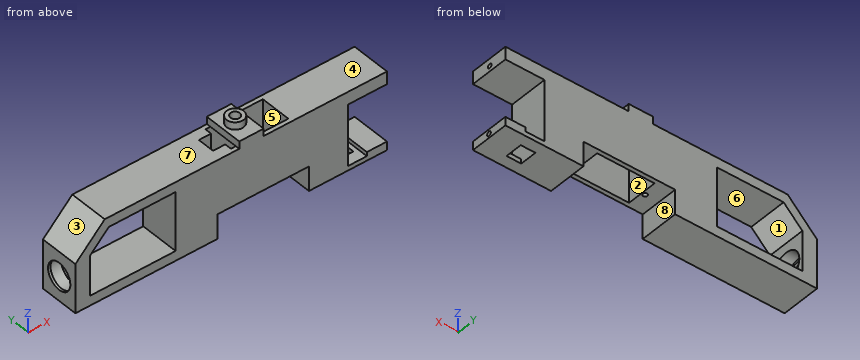
from build123d import *

# Parameters (mm, degrees)
BOSS_EXTRUDE1_DEPTH      = 8
BOSS_EXTRUDE1_DEPTH_BACK = 8
SKETCH2_R                = 5.5
CUT_EXTRUDE1_DEPTH       = 8
CUT_EXTRUDE2_DEPTH       = 16
SKETCH4_R                = 6.5
CUT_EXTRUDE3_DEPTH       = 5
SKETCH5_W                = 23.5
SKETCH5_H                = 12.6
CUT_EXTRUDE4_DEPTH       = 33
SKETCH6_R                = 0.9
CUT_EXTRUDE5_DEPTH       = 17
SKETCH7_W                = 6
SKETCH7_H                = 7
CUT_EXTRUDE6_DEPTH       = 7
SKETCH8_W                = 5
SKETCH8_H                = 7
CUT_EXTRUDE7_DEPTH       = 10
SKETCH9_R                = 0.899999999
CUT_EXTRUDE8_DEPTH       = 7
SKETCH10_W               = 37.5
SKETCH10_H               = 16
CUT_EXTRUDE9_DEPTH       = 10
SKETCH11_W               = 10
SKETCH11_H               = 16
BOSS_EXTRUDE2_DEPTH      = 3
SKETCH12_R               = 3.5
SKETCH12_R_2             = 1.9
BOSS_EXTRUDE3_DEPTH      = 3
SKETCH13_R               = 1.9
CUT_EXTRUDE10_DEPTH      = 3


with BuildPart() as part:
    # Sketch1 → Boss-Extrude1 (new body, two sides)
    with BuildSketch(Plane(origin=(0, 0, 0), x_dir=(1, 0, 0), z_dir=(0, 1, 0))) as boss_extrude1_sk:
        Polygon((64, -16.835969506), (47.993540801, -16.835969506), (47.993540801, 8.164030494), (55.763890835, 8.164030494), (55.763890835, 6.5), (64, 6.5), (64, 10), (-63.5, 10), (-63.5, -10), (-51.5, -22), (64, -22), align=None)
    extrude(amount=BOSS_EXTRUDE1_DEPTH)
    extrude(boss_extrude1_sk.sketch, amount=-BOSS_EXTRUDE1_DEPTH_BACK)

    # Sketch2 → Cut-Extrude1 (cut)
    with BuildSketch(Plane.ZY.offset(63.5)):
        Circle(SKETCH2_R)
    extrude(amount=-CUT_EXTRUDE1_DEPTH, mode=Mode.SUBTRACT)

    # Sketch3 → Cut-Extrude2 (cut)
    with BuildSketch(Plane(origin=(0, 8, 0), x_dir=(1, 0, 0), z_dir=(0, 1, 0))):
        Polygon((-57.5, 6), (-22.5, 6), (-22.5, -18), (-49.843145751, -18), (-57.5, -10.343145751), align=None)
    extrude(amount=-CUT_EXTRUDE2_DEPTH, mode=Mode.SUBTRACT)

    # Sketch4 → Cut-Extrude3 (cut)
    with BuildSketch(Plane(origin=(-57.5, 0, 0), x_dir=(0, 0, -1), z_dir=(1, 0, 0))):
        Circle(SKETCH4_R)
    extrude(amount=-CUT_EXTRUDE3_DEPTH, mode=Mode.SUBTRACT)

    # Sketch5 → Cut-Extrude4 (cut, through all)
    with BuildSketch(Plane(origin=(0, 0, -10), x_dir=(-1, 0, 0), z_dir=(0, 0, -1))):
        with Locations((-13.3, 0)):
            Rectangle(SKETCH5_W, SKETCH5_H)
    extrude(amount=-CUT_EXTRUDE4_DEPTH, mode=Mode.SUBTRACT)

    # Sketch6 → Cut-Extrude5 (cut)
    with BuildSketch(Plane(origin=(0, 0, -10), x_dir=(-1, 0, 0), z_dir=(0, 0, -1))):
        with Locations((-0.2, 0)):
            Circle(SKETCH6_R)
        with Locations((-27.5, 0)):
            Circle(SKETCH6_R)
    extrude(amount=-CUT_EXTRUDE5_DEPTH, mode=Mode.SUBTRACT)

    # Sketch7 → Cut-Extrude6 (cut)
    with BuildSketch(Plane(origin=(0, 0, -10), x_dir=(-1, 0, 0), z_dir=(0, 0, -1))):
        with Locations((-50.993540801, 0)):
            Rectangle(SKETCH7_W, SKETCH7_H)
    extrude(amount=-CUT_EXTRUDE6_DEPTH, mode=Mode.SUBTRACT)

    # Sketch8 → Cut-Extrude7 (cut)
    with BuildSketch(Plane.XY.offset(22)):
        with Locations((-0.95, 0)):
            Rectangle(SKETCH8_W, SKETCH8_H)
    extrude(amount=-CUT_EXTRUDE7_DEPTH, mode=Mode.SUBTRACT)

    # Sketch9 → Cut-Extrude8 (cut)
    with BuildSketch(Plane(origin=(64, 0, 0), x_dir=(0, 0, -1), z_dir=(1, 0, 0))):
        with Locations((-18.998394534, 0.246992199)):
            Circle(SKETCH9_R)
        with Locations((8.299298665, -0.107896588)):
            Circle(SKETCH9_R)
    extrude(amount=-CUT_EXTRUDE8_DEPTH, mode=Mode.SUBTRACT)

    # Sketch10 → Cut-Extrude9 (cut)
    with BuildSketch(Plane(origin=(0, 0, -10), x_dir=(-1, 0, 0), z_dir=(0, 0, -1))):
        with Locations((-13.3, 0)):
            Rectangle(SKETCH10_W, SKETCH10_H)
    extrude(amount=-CUT_EXTRUDE9_DEPTH, mode=Mode.SUBTRACT)

    # Sketch11 → Boss-Extrude2 (add)
    with BuildSketch(Plane.XY.offset(22)):
        with Locations((8.55, 0)):
            Rectangle(SKETCH11_W, SKETCH11_H)
    extrude(amount=BOSS_EXTRUDE2_DEPTH)

    # Sketch12 → Boss-Extrude3 (add)
    with BuildSketch(Plane.XY.offset(25)):
        with Locations((8.499999912, 0)):
            Circle(SKETCH12_R)
        with Locations((8.499999912, 0)):
            Circle(SKETCH12_R_2, mode=Mode.SUBTRACT)
    extrude(amount=BOSS_EXTRUDE3_DEPTH)

    # Sketch13 → Cut-Extrude10 (cut)
    with BuildSketch(Plane.XY.offset(25)):
        with Locations((8.499999912, 0)):
            Circle(SKETCH13_R)
    extrude(amount=-CUT_EXTRUDE10_DEPTH, mode=Mode.SUBTRACT)


solid = part.part
Geometry check sheet. Reference: the model listing, model coordinates, mm. Face numbers are marked on the shaded views. A direction names the side the tool comes from. Round coordinates to 2 decimals unless told otherwise and drop trailing zeros. Order: outer loops, then holes, each group sorted by start corner. A loop starts at its lowest first (then second) coordinate and runs counter-clockwise, first axis right, second up. Notation, with made-up numbers: (89.25, 44.25) - (94.25, 44.25) arc R33 ccw to (94.25, 80.25) - close; hole circle Ø11 at (46.5, 48.5). An arc over 180 degrees is marked (long way). One line per question, with ' | ' between items. Start each with the question number.
(1) Sectioned sample at D-D on x = 8.5. Record the cut outline in (y, z), and give its area (3 significant figures).
(2) Sectioned sample at C-C on z = -2.5. Record the cut outline in (x, y), and give its area (3 significant figures).
(3) Thickness scan on L1, parallel to Y at x = -63.2, z = 0; L2, parallel to X at y = 1.25, z = 4; L3, parallel to Z at x = -26.5, y = -2.25. Record the ranges inside material, lowest first. Write a range as [from, to].
(4) Release check for a two-part mould opening along X. For the marked faces 1, 2, 3 and 4 record: released by +X, released by -X, zero draft, split by the parting line, or undercut.
(5) Sectioned sample at B-B on x = -44. Record the cut outline in (y, z).
(6) Access from +Z, -Z, +X, -X, +Y, -Y to the whole of each face (thin tool, end or side, straight path). Record for the marked faces 5, 6, 7 and 8.
(7) Sectioned sample at A-A on z = 8.5. Record the cut outline in (x, y), and give its area (3 significant figures).
(8) Depth check by flat-ended pin: pin 1 Ø6 at (y, z) = (-4, 7) entering from +X; pin 2 Ø6 at (x, y) = (-42.5, -3.5) entering from +Z; pin 3 Ø2 at (x, y) = (5, 4) entering from +Z. Enter the tip coordinate at first touch or a pass-through.
Conclusion:
1) outline: (-8, 0) - (-6.3, 0) - (-6.3, 22) - (-1.9, 22) - (-1.9, 28) - (-3.5, 28) - (-3.5, 25) - (-8, 25) - close; (1.9, 22) - (6.3, 22) - (6.3, 0) - (8, 0) - (8, 25) - (3.5, 25) - (3.5, 28) - (1.9, 28) - close | area: 121 mm2
2) outline: (-63.5, -8) - (-57.5, -8) - (-57.5, -6) - (-62.5, -6) - (-62.5, -4.9) - (-63.5, -4.9) - close; (-63.5, 4.9) - (-62.5, 4.9) - (-62.5, 6) - (-57.5, 6) - (-57.5, 8) - (-63.5, 8) - close; (-22.5, -8) - (-5.45, -8) - (-5.45, 8) - (-22.5, 8) - close; (32.05, -8) - (47.99, -8) - (47.99, 8) - (32.05, 8) - close | area: 554 mm2
3) L1: y = [-8, -5.5], [5.5, 8] | L2: x = [-22.5, 1.55], [25.05, 47.99] | L3: z = [-10, -6], [18, 22]
4) face 1: undercut | face 2: undercut | face 3: released by -X | face 4: zero draft
5) outline: (-8, -10) - (8, -10) - (8, -6) - (-8, -6) - close; (-8, 18) - (8, 18) - (8, 22) - (-8, 22) - close
6) face 5: +Z, -Z | face 6: +Y, -Y | face 7: +Z, -X, +Y, -Y | face 8: -Z, +Y, -Y
7) outline: (-63.5, -8) - (-57.5, -8) - (-57.5, 8) - (-63.5, 8) - close; (-22.5, -8) - (47.99, -8) - (47.99, 8) - (-22.5, 8) - close; hole (1.55, -6.3) - (25.05, -6.3) - (25.05, 6.3) - (1.55, 6.3) - close | area: 928 mm2
8) pin 1: stops at x = 47.99 | pin 2: stops at z = 22 | pin 3: stops at z = 25
